Read the model definition and answer for the solid it produces. Units are mm, in the model's axes. Face numbers are marked on the shaded views. A direction names the side the tool comes from. Coordinates: 2 decimals unless noted, no trailing zeros. Loops run counter-clockwise (first coordinate to the right, second up) from the corner with the lowest first, then second, coordinate; pieces in that order, holes last. Notation, with made-up numbers: M 69,-13.5 L 94,-13.5 A7 cw 94,-9.5 Z; hole C 80,-26.5 d10. An arc over 180 degrees is marked long. Put each result on its own line as item: value.
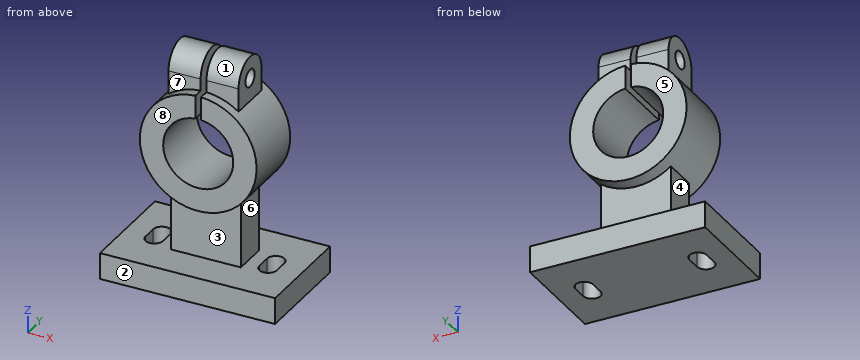
from build123d import *

# Parameters (mm, degrees)
F0_R      = 40
F0_R_2    = 24
F1_DEPTH  = 22
F2_W      = 48
F2_H      = 64
F3_DEPTH  = 12
F4_W      = 120
F4_H      = 72
F5_DEPTH  = 18
F7_DEPTH  = 24
F8_R      = 6
F9_DEPTH  = 84.001
F11_DEPTH = 25
F12_W     = 4
F12_H     = 50
F13_DEPTH = 25


# Not quite as in the source:
# - a pattern or mirror of a feature is missing from the dataset's text; its kind, count and spacing are read off the source's solid


with BuildPart() as f1:
    # F0 (on Front) → F1 (new body, symmetric)
    with BuildSketch(Plane.XZ):
        Circle(F0_R)
        Circle(F0_R_2, mode=Mode.SUBTRACT)
    extrude(amount=F1_DEPTH, both=True)

    # F2 (on Front) → F3 (join, symmetric)
    with BuildSketch(Plane.XZ):
        with Locations((0, -64)):
            Rectangle(F2_W, F2_H)
    extrude(amount=F3_DEPTH, both=True)

    # F4 (on face) → F5 (join)
    with BuildSketch(Plane(origin=(0, 0, -96), x_dir=(1, 0, 0), z_dir=(0, 0, -1))):
        Rectangle(F4_W, F4_H)
    extrude(amount=-F5_DEPTH)

    # F6 (on Right) → F7 (join, symmetric)
    with BuildSketch(Plane.YZ):
        with BuildLine():
            Line((-15, 25), (15, 25))
            Line((15, 25), (15, 48))
            ThreePointArc((15, 48), (0, 63), (-15, 48))
            Line((-15, 48), (-15, 25))
        make_face()
    extrude(amount=F7_DEPTH, both=True)

    # F8 (on face) → F9 (cut, through all)
    with BuildSketch(Plane.YZ.offset(24)):
        with Locations((0, 48)):
            Circle(F8_R)
    extrude(amount=-F9_DEPTH, mode=Mode.SUBTRACT)

    # F10 (on face) → F11 (cut)
    with BuildSketch(Plane(origin=(0, 0, -96), x_dir=(1, 0, 0), z_dir=(0, 0, -1))):
        with BuildLine():
            Line((45, -5), (45, 5))
            ThreePointArc((45, 5), (39, 11), (33, 5))
            Line((33, 5), (33, -5))
            ThreePointArc((33, -5), (39, -11), (45, -5))
        make_face()
    f11 = extrude(amount=-F11_DEPTH, mode=Mode.SUBTRACT)

    # F11_copies: F11 across plane
    add(f11.mirror(Plane(origin=(0, 0, 0), x_dir=(0, 0, -1), z_dir=(-1, 0, 0))), mode=Mode.SUBTRACT)

    # F12 (on Front) → F13 (cut, symmetric)
    with BuildSketch(Plane.XZ):
        with Locations((0, 45)):
            Rectangle(F12_W, F12_H)
    extrude(amount=F13_DEPTH, both=True, mode=Mode.SUBTRACT)


solid = f1.part
1) Given pin 1 Ø17.5 at (x, z) = (8.5, 37.5) entering from -Y; pin 2 Ø19 at (y, z) = (0, 48) entering from -X; pin 3 Ø17.5 at (x, z) = (13, 39.5) entering from +Y, each flat-ended and moving along its own axis, determine where each tip first touches the part or whether it passes through.
Answer list:
pin 1: stops at y = -22
pin 2: stops at x = -24
pin 3: stops at y = 22
2) Find section D-D, the plane z = 0. Write down the section's boundary in (x, y), plus the area to 3 significant figures.
Answer list:
outline: M -40,-22 L -24,-22 L -24,22 L -40,22 Z; M 24,-22 L 40,-22 L 40,22 L 24,22 Z
area: 1,410 mm^2
3) Which of the six approach directions +Z, -Z, +X, -X, +Y, -Y give full straight-line access (tool end or side, diameter ignored) to the marked faces 4, 5, 6, 7 and 8?
Answer list:
face 4: -X, +Y, -Y
face 5: +Z, +X, -X, +Y
face 6: +X, +Y, -Y
face 7: +Z, -X, -Y
face 8: +Z, +X, -X, -Y
4) Straight lines are drawn through the part: line 1 (X direction, y = 8, z = 0); line 2 (Z direction, x = -18.75, y = 0); line 3 (Z direction, x = -10.5, y = 0). For each, find the intervals that lie inside material, in ascending order. Write a range as [from, to].
Answer list:
line 1: x = [-40, -24], [24, 40]
line 2: z = [-96, -14.98], [14.98, 42], [54, 63]
line 3: z = [-96, -21.58], [21.58, 42], [54, 63]
5) Find section C-C, the plane y = 0. Count the separate pieces of the cut face and the enclosed holes in it, plus the area to 3 significant figures.
Answer list:
separate pieces: 5
enclosed holes: 0
area: 7,430 mm^2
6) Find section A-A, the plane y = -19.5. Write down the section's boundary in (x, z), plus the area to 3 significant figures.
Answer list:
outline: M -60,-96 L 60,-96 L 60,-78 L -60,-78 Z; M -2,23.92 L -2,39.95 A40 ccw long 2,39.95 L 2,23.92 A24 cw long Z
area: 5,310 mm^2
7) Find section B-B, the plane x = -16. Write down the section's boundary in (y, z), plus the area to 3 significant figures.
Answer list:
outline: M -36,-96 L 36,-96 L 36,-78 L 12,-78 L 12,-36.66 L 22,-36.66 L 22,-17.89 L -22,-17.89 L -22,-36.66 L -12,-36.66 L -12,-78 L -36,-78 Z; M -22,17.89 L 22,17.89 L 22,36.66 L 15,36.66 L 15,48 A15 ccw -15,48 L -15,36.66 L -22,36.66 Z; hole C 0,48 d12
area: 4,520 mm^2
8) Determine the mould class of the marked faces 1, 2 and 3 for opening direction Z: released by +Z, released by -Z, zero draft, split by the parting line, or undercut.
Answer list:
face 1: released by +Z
face 2: zero draft
face 3: undercut
